```python
from build123d import *

# Parameters (mm, degrees)
SKETCH1_W             = 76.2
SKETCH1_H             = 76.2
BOSS_EXTRUDE1_DEPTH   = 3.175
SKETCH2_W             = 69.79412
SKETCH2_H             = 69.79412
BOSS_EXTRUDE2_DEPTH   = 9.525
F_6_32_TAPPED_HOLE1_D = 2.7051
CIRPATTERN1_COUNT     = 4
SKETCH14_R            = 3.175
CUT_EXTRUDE1_DEPTH    = 56.358016583
SKETCH15_W            = 50.74412
SKETCH15_H            = 26.95956
CUT_EXTRUDE2_DEPTH    = 9.525
FILLET1_R             = 12.7
FILLET1_OF_MIRROR3_R  = 12.7


with BuildPart() as part:
    # Sketch1 → Boss-Extrude1 (new body)
    with BuildSketch(Plane(origin=(0, 0, 0), x_dir=(1, 0, 0), z_dir=(0, 1, 0))):
        Rectangle(SKETCH1_W, SKETCH1_H)
    extrude(amount=BOSS_EXTRUDE1_DEPTH)

    # Sketch2 → Boss-Extrude2 (add)
    with BuildSketch(Plane(origin=(0, 3.175, 0), x_dir=(1, 0, 0), z_dir=(0, 1, 0))):
        Rectangle(SKETCH2_W, SKETCH2_H)
    extrude(amount=BOSS_EXTRUDE2_DEPTH)

    # Sketch9 → 4-40 Tapped Hole1 (revolve, cut)
    with BuildSketch(Plane(origin=(34.89706, 7.9375, 12.7), x_dir=(0, 0, -1), z_dir=(0, 1, 0))):
        Polygon((0, 0), (0, 7.283152758), (1.1303, 6.604), (1.1303, 0), align=None)
    f_4_40_tapped_hole1 = revolve(axis=Axis((41.24706, 7.9375, 12.7), (-1, 0, 0)), mode=Mode.SUBTRACT)

    # Mirror1: 4-40 Tapped Hole1 across plane
    add(f_4_40_tapped_hole1.mirror(Plane.XY), mode=Mode.SUBTRACT)

    # Mirror2: 4-40 Tapped Hole1 across plane
    add(f_4_40_tapped_hole1.mirror(Plane(origin=(0, 0, 0), x_dir=(0, 0, 1), z_dir=(1, 0, 0))), mode=Mode.SUBTRACT)

    # Mirror2 copy 1 sketch → Mirror2 copy 1 (revolve, cut)
    with BuildSketch(Plane(origin=(-34.89706, 7.9375, -12.7), x_dir=(0, 0, 1), z_dir=(0, 1, 0))):
        Polygon((0, 0), (0, 7.283152758), (1.1303, 6.604), (1.1303, 0), align=None)
    revolve(axis=Axis((-41.24706, 7.9375, -12.7), (1, 0, 0)), mode=Mode.SUBTRACT)

    # 6-32 Tapped Hole1 (through all)
    with Locations(Plane(origin=(0, 0, 0), x_dir=(-1, 0, 0), z_dir=(0, -1, 0))):
        with Locations((-32.5501, 32.5501)):
            f_6_32_tapped_hole1 = Hole(F_6_32_TAPPED_HOLE1_D / 2)

    # CirPattern1: 6-32 Tapped Hole1 ×4 about axis
    cirpattern1_axis = Axis((0, 0, 0), (0, 1, 0))
    for i in range(1, CIRPATTERN1_COUNT):
        add(f_6_32_tapped_hole1.rotate(cirpattern1_axis, i * 360 / CIRPATTERN1_COUNT), mode=Mode.SUBTRACT)

    # Sketch14 → Cut-Extrude1 (cut, through all)
    with BuildSketch(Plane.XZ):
        with Locations(Location((0, 0, 0), (0, 0, 270))):
            Circle(SKETCH14_R)
    extrude(amount=-CUT_EXTRUDE1_DEPTH, mode=Mode.SUBTRACT)

    # Sketch15 → Cut-Extrude2 (cut)
    with BuildSketch(Plane(origin=(0, 12.7, 0), x_dir=(1, 0, 0), z_dir=(0, 1, 0))):
        with Locations((0, -21.41728)):
            Rectangle(SKETCH15_W, SKETCH15_H)
    cut_extrude2 = extrude(amount=-CUT_EXTRUDE2_DEPTH, mode=Mode.SUBTRACT)

    # Fillet1
    fillet1_edges = [part.edges().sort_by_distance(p)[0] for p in [
        (-25.37206, 7.9375, 7.9375),
        (25.37206, 7.9375, 7.9375),
    ]]
    fillet(fillet1_edges, radius=FILLET1_R)

    # Sketch17 → 6-32 Tapped Hole2 (revolve, cut)
    with BuildSketch(Plane(origin=(0, 7.9375, 7.9375), x_dir=(0, -1, 0), z_dir=(1, 0, 0))):
        Polygon((0, 0), (0, 10.46469403), (1.35255, 9.652), (1.35255, 0), align=None)
    f_6_32_tapped_hole2 = revolve(axis=Axis((0, 7.9375, 14.2875), (0, 0, -1)), mode=Mode.SUBTRACT)

    # Mirror3: Cut-Extrude2, 6-32 Tapped Hole2 across plane
    add(cut_extrude2.mirror(Plane.XY), mode=Mode.SUBTRACT)
    add(f_6_32_tapped_hole2.mirror(Plane.XY), mode=Mode.SUBTRACT)

    # Fillet1 of Mirror3
    fillet1_of_mirror3_edges = [part.edges().sort_by_distance(p)[0] for p in [
        (-25.37206, 7.9375, -7.9375),
        (25.37206, 7.9375, -7.9375),
    ]]
    fillet(fillet1_of_mirror3_edges, radius=FILLET1_OF_MIRROR3_R)


solid = part.part
```
Input: part model. Units: mm. Frame: model coordinates. A direction names the side the tool comes from. Give positions to 0.01 mm unless a question says otherwise; leave off trailing zeros. Loops run counter-clockwise (first coordinate to the right, second up) from the corner with the lowest first, then second, coordinate; pieces in that order, holes last.
1) Section query A-A on x = 0. Return the cut outline in (y, z) (1 decimal), and give its area (3 significant figures).
A:
outline: (0, -38.1) - (3.2, -38.1) - (3.2, -7.9) - (6.6, -7.9) - (6.6, -3.2) - (0, -3.2) - close; (0, 3.2) - (6.6, 3.2) - (6.6, 7.9) - (3.2, 7.9) - (3.2, 38.1) - (0, 38.1) - close; (9.3, -7.9) - (12.7, -7.9) - (12.7, -3.2) - (9.3, -3.2) - close; (9.3, 3.2) - (12.7, 3.2) - (12.7, 7.9) - (9.3, 7.9) - close
area: 287 mm2
2) Line query: L1, parallel to X at y = 11.25, z = -26; L2, parallel to Y at x = -32.25, z = 12.7; L3, parallel to Y at x = 0, z = 6.45. Output: solid intervals per line, ascending.
A:
L1: x = -34.9 to -25.37, 25.37 to 34.9
L2: y = 0 to 6.81, 9.07 to 12.7
L3: y = 0 to 6.58, 9.29 to 12.7
3) Contact query for flat-ended pins moving along their axis: pin 1 (3.5 mm diameter, centred on y = 7.94, z = 12.7, fed in from -X); pin 2 (3.5 mm diameter, centred on y = 7.94, z = -12.7, fed in from +X); pin 3 (4 mm diameter, centred on x = -4.5, y = 10, fed in from +Z); pin 4 (2 mm diameter, centred on x = 32.55, z = 32.55, fed in from -Y). Output: stop coordinate, or through.
A:
pin 1: stops at x = -34.9
pin 2: stops at x = 34.9
pin 3: stops at z = 7.94
pin 4: passes through
4) Reachability of faces 1 (the cylindrical face through (21.553, 7.871, -11.559)), 2 (the flat face through (0, 10, 7.938)), 3 (the cylindrical face through (-31.641, 8.625, 13.597)) from +Z, -Z, +X, -X, +Y, -Y: full face, straight path, thin tool, end or side. Return the list, or none.
A:
face 1: -Z, +Y
face 2: +Z, +Y
face 3: -X
5) Section query B-B on z = 0. Return the cut outline in (x, y) (3 decimals).
A:
outline: (-38.1, 0) - (-3.175, 0) - (-3.175, 12.7) - (-34.897, 12.7) - (-34.897, 3.175) - (-38.1, 3.175) - close; (3.175, 0) - (38.1, 0) - (38.1, 3.175) - (34.897, 3.175) - (34.897, 12.7) - (3.175, 12.7) - close
6) Mould query, pull axis X, two halves, no side actions, for faces 4 (the conical face through (-27.73, 8.11, 12.61)), 5 (the flat face through (-25.372, 8, 28)), 6 (the flat face through (-30, 8, -34.897)). Classes: released by +X, released by -X, zero draft, split by the parting line, or undercut.
A:
face 4: released by -X
face 5: undercut
face 6: zero draft
7) Section query C-C on z = -29. Return the cut outline in (x, y) (3 decimals).
A:
outline: (-38.1, 0) - (38.1, 0) - (38.1, 3.175) - (34.897, 3.175) - (34.897, 12.7) - (25.372, 12.7) - (25.372, 3.175) - (-25.372, 3.175) - (-25.372, 12.7) - (-34.897, 12.7) - (-34.897, 3.175) - (-38.1, 3.175) - close
8) Section query D-D on y = 5. Count the separate pieces of the cut face and the enclosed holes in it, and give its area (3 significant figures).
A:
separate pieces: 1
enclosed holes: 5
area: 2,220 mm2
